Geometry: final body of the model. Coordinates: model frame, mm. Face numbers are marked on the shaded views. Round coordinates to 2 decimals unless told otherwise and drop trailing zeros. Order: outer loops, then holes, each group sorted by start corner. A loop starts at its lowest first (then second) coordinate and runs counter-clockwise, first axis right, second up. Notation, with made-up numbers: M -10.75,46 L 40.25,46 A26 cw 40.25,83 Z; hole C -17,-21.5 d2. An arc over 180 degrees is marked long. Return JSON: item names as keys, results as strings. Group by question number.
Q1. Mould query, pull axis Z, two halves, no side actions, for the marked faces 1, 2 and 3. Classes: released by +Z, released by -Z, zero draft, split by the parting line, or undercut.
Q2. Cut plane D-D on y = 10. Output: boundary loops of the cut face in (x, z), and give its area (3 significant figures).
Q3. Ray query, probe 1 along X at (y, z) = (10, -3.25); probe 2 along Z at (x, y) = (1, 0); probe 3 along Y at (x, z) = (1.5, 5.5). Return the intervals inside material, ascending.
Q4. Contact query for flat-ended pins moving along their axis: pin 1 (1 mm diameter, centred on x = -9.5, y = -10, fed in from -Z); pin 2 (4 mm diameter, centred on x = 13.5, y = 10.5, fed in from +Z); pin 3 (8 mm diameter, centred on x = 14.5, y = -6, fed in from -Z); pin 4 (8 mm diameter, centred on x = -9, z = 1, fed in from -Y). Output: stop coordinate, or through.
Q5. Cut plane A-A on y = 0. Output: boundary loops of the cut face in (x, z), and give its area (3 significant figures).
Q6. Cut plane B-B on x = 15. Output: boundary loops of the cut face in (y, z).
Q7. Cut plane C-C on z = 1. Output: boundary loops of the cut face in (x, y).
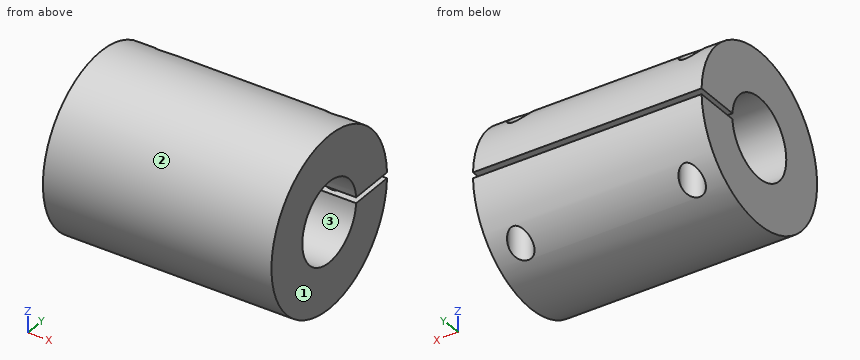
Autodesk Inventor part; units mm, degrees
ref_plane "Work Plane1" through (0, 15, 0) normal (0, 1, 0) x (-1, 0, 0)
ref_plane "Work Plane2" through (0, 0, -15) normal (0, 0, 1) x (1, 0, 0)
ref_plane "YZ Plane" through (0, 0, 0) normal (1, 0, 0) x (0, 1, 0)
sketch "Sketch1" plane through (0, 0, 0) normal (1, 0, 0) x (0, 1, 0)
  circle A0 centre (0, 0) radius 7
  circle A1 centre (0, 0) radius 15
  dimension "d0" = 14
  dimension "d1" = 30
extrude "Extrusion1" add sketch "Sketch1" along normal blind 20 and the other way blind 20
ref_plane "Work Plane1" through (0, 15, 0) normal (0, 1, 0) x (-1, 0, 0)
sketch "Sketch3" plane through (0, 15, 0) normal (0, 1, 0) x (-1, 0, 0)
  line L0 (-20, 0) -> (20, 0) construction
  line L1 (-20, 15) -> (-20, -15)
  line L2 (20, 7) -> (20, -7)
  line L3 (-20, 0.5) -> (20, 0.5)
  line L4 (20, 0.5) -> (20, -0.5)
  line L5 (20, -0.5) -> (-20, -0.5)
  line L6 (-20, -0.5) -> (-20, 0.5)
  point P0 (0, 0)
  dimension "d10" = 0.5
  dimension "d11" = 0.5
extrude "Extrusion2" cut sketch "Sketch3" against normal up to next
ref_plane "Work Plane2" through (0, 0, -15) normal (0, 0, 1) x (1, 0, 0)
sketch "Sketch4" plane through (0, 0, -15) normal (0, 0, 1) x (1, 0, 0)
  line L0 (-20, -7) -> (-20, 6.9821) construction
  line L1 (-20, 0) -> (20, 0) construction
  line L2 (20, 6.9821) -> (20, -7) construction
  circle A0 centre (-15, 10) radius 2
  line L3 (-20, 14.9917) -> (20, 14.9917) construction
  line L4 (0, 14.9917) -> (0, -15) construction
  line L5 (-20, -15) -> (20, -15) construction
  circle A1 centre (15, 10) radius 2
  point P0 (0, 0)
  dimension "d14" = 10
  dimension "d15" = 15
  dimension "d16" = 4
extrude "Extrusion3" cut sketch "Sketch4" along normal through all
properties part number "14mm_shaft_coupler"
Result sheet:
{
 "1": {"face 1": "zero draft", "face 2": "split by the parting line", "face 3": "undercut"},
 "2": {"outline": "M -20,-11.18 L -17,-11.18 L -17,-0.5 L -20,-0.5 Z; M -20,0.5 L -17,0.5 L -17,11.18 L -20,11.18 Z; M -13,-11.18 L 13,-11.18 L 13,-0.5 L -13,-0.5 Z; M -13,0.5 L 13,0.5 L 13,11.18 L -13,11.18 Z; M 17,-11.18 L 20,-11.18 L 20,-0.5 L 17,-0.5 Z; M 17,0.5 L 20,0.5 L 20,11.18 L 17,11.18 Z", "area": "684 mm²"},
 "3": {"probe 1": "x = -20 to -17, -13 to 13, 17 to 20", "probe 2": "z = -15 to -7, 7 to 15", "probe 3": "y = -13.96 to -4.33, 4.33 to 13.96"},
 "4": {"pin 1": "stops at z = -11.61", "pin 2": "stops at z = 12.36", "pin 3": "stops at z = -14.87", "pin 4": "stops at y = -15"},
 "5": {"outline": "M -20,-15 L 20,-15 L 20,-7 L -20,-7 Z; M -20,7 L 20,7 L 20,15 L -20,15 Z", "area": "640 mm²"},
 "6": {"outline": "M 6.98,-0.5 A7 cw long 6.98,0.5 L 8,0.5 L 8,12.69 A15 ccw long 8,-12.69 L 8,-0.5 Z; M 12,-9 A15 ccw 14.99,-0.5 L 12,-0.5 Z; M 12,0.5 L 14.99,0.5 A15 ccw 12,9 Z"},
 "7": {"outline": "M -20,-14.97 L 20,-14.97 L 20,-6.93 L -20,-6.93 Z; M -20,6.93 L 20,6.93 L 20,14.97 L -20,14.97 Z; hole C -15,10 d4; hole C 15,10 d4"}
}
